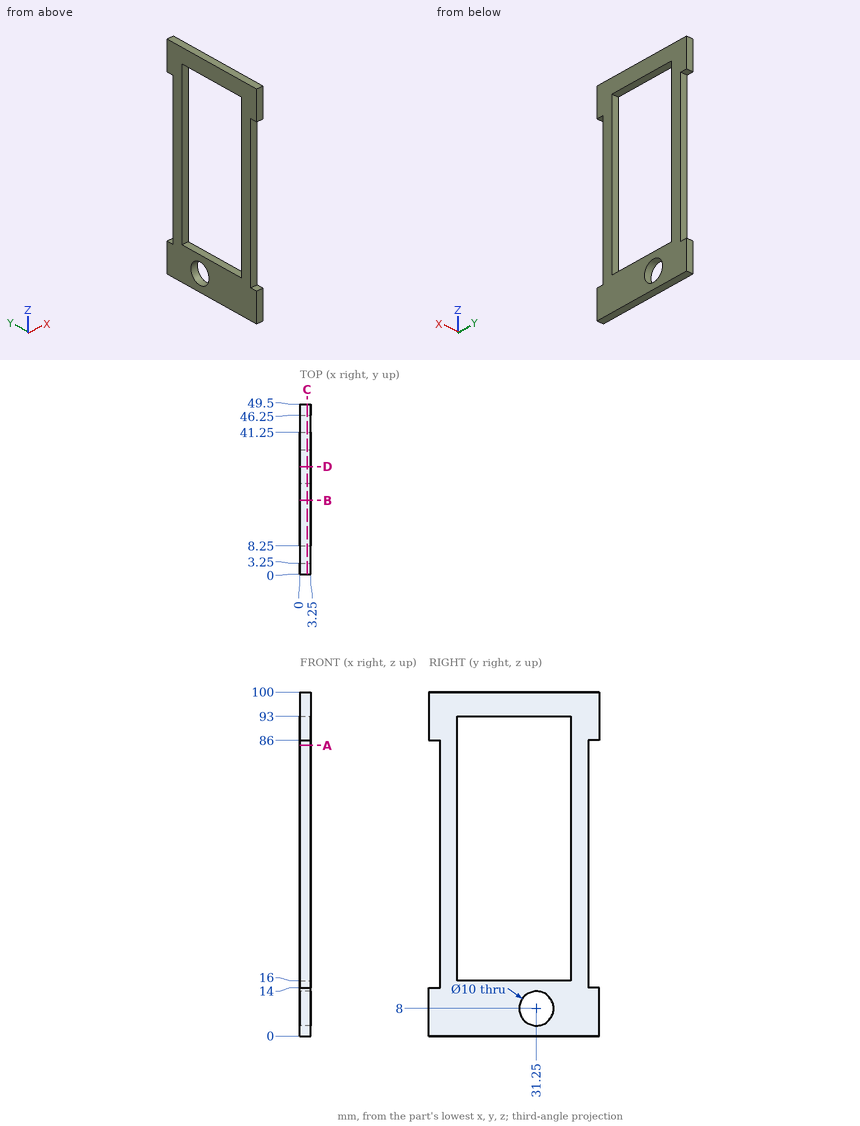
Study the drawing (mm; zero at the part's minimum x, y, z) and answer. Coordinates: 2 decimals unless noted, no trailing zeros. Write each loop counter-clockwise with the first axis right and the second up, starting at its lowest first coordinate (ties: lowest second). Pieces come first, ordered by that corner, then holes. Notation, with made-up numbers: (40, -40) - (62, -40) arc R8 cw to (62, -30) - close; hole circle Ø11 at (-34, -33.5). An arc over 180 degrees is marked (long way). One line per question, with ' | ' between items.
1) Consider probe 1 along Z at (x, y) = (2.5, 31.25); probe 2 along Z at (x, y) = (1.9, 12); probe 3 along Z at (x, y) = (2.3, 34.5). Determine where each line is inside the solid, lowest interval first. Write a range as [from, to].
Checks:
probe 1: [0, 3], [13, 16], [93, 100] | probe 2: [0, 16], [93, 100] | probe 3: [0, 4.2], [11.8, 16], [93, 100]
2) Flat-ended cylindrical pins translate along their axes: P1, Ø1.6, axis at x = 1.5, z = 48, coming from the +Y side; P2, Ø1, axis at x = 2.5, z = 61, coming from the -Y side. Find the tip coordinate at first contact, or state that the pin passes through.
Checks:
P1: y = 46.25 | P2: y = 3.25
3) Find section C-C, the plane x = 2.15. Determine the outline of the cut face in (y, z).
Checks:
outline: (0, 0) - (49.5, 0) - (49.5, 14) - (46.25, 14) - (46.25, 86) - (49.5, 86) - (49.5, 100) - (0, 100) - (0, 86) - (3.25, 86) - (3.25, 14) - (0, 14) - close; hole (8.25, 16) - (41.25, 16) - (41.25, 93) - (8.25, 93) - close; hole circle Ø10 at (31.25, 8)
4) Find section A-A, the plane z = 84.5. Determine the outline of the cut face in (x, y), and give its area (3 significant figures).
Checks:
outline: (0, 3.25) - (3.25, 3.25) - (3.25, 8.25) - (0, 8.25) - close; (0, 41.25) - (3.25, 41.25) - (3.25, 46.25) - (0, 46.25) - close | area: 32.5 mm2
5) Find section D-D, the plane y = 31.25. Determine the outline of the cut face in (x, z).
Checks:
outline: (0, 0) - (3.25, 0) - (3.25, 3) - (0, 3) - close; (0, 13) - (3.25, 13) - (3.25, 16) - (0, 16) - close; (0, 93) - (3.25, 93) - (3.25, 100) - (0, 100) - close
6) Find section B-B, the plane y = 21.5. Determine the outline of the cut face in (x, z).
Checks:
outline: (0, 0) - (3.25, 0) - (3.25, 16) - (0, 16) - close; (0, 93) - (3.25, 93) - (3.25, 100) - (0, 100) - close
